Read the model definition and answer for the solid it produces. Units are mm, in the model's axes. A direction names the side the tool comes from. Give positions to 0.01 mm unless a question says otherwise; leave off trailing zeros. Order: outer loops, then holes, each group sorted by start corner. A loop starts at its lowest first (then second) coordinate and runs counter-clockwise, first axis right, second up. Notation, with made-up numbers: (56.25, 51) -> (67.25, 51) arc R7 cw to (67.25, 60) -> close; hole circle Ø9 at (79.5, -2.5). An arc over 180 degrees is marked (long way). One line per question, with ' | ' between items. Start each with the question number.
```python
from build123d import *

# Parameters (mm, degrees)
SKETCH1_W           = 51.225
SKETCH1_H           = 33.05
BOSS_EXTRUDE1_DEPTH = 6.35
SKETCH7_R           = 11.05
SKETCH7_R_2         = 3.556
CUT_EXTRUDE3_DEPTH  = 4.7625
SKETCH8_R           = 1.25
CUT_EXTRUDE4_DEPTH  = 15
FILLET3_R           = 5.08
CHAMFER2_SIZE       = 0.2


with BuildPart() as part:
    # Sketch1 → Boss-Extrude1 (new body)
    with BuildSketch(Plane.XY.offset(152.111703917)):
        with Locations((-7.6125, 2.525)):
            Rectangle(SKETCH1_W, SKETCH1_H)
    extrude(amount=-BOSS_EXTRUDE1_DEPTH)

    # Sketch7 → Cut-Extrude3 (cut)
    with BuildSketch(Plane.XY.offset(152.111703917)):
        Circle(SKETCH7_R)
        with Locations((-22.225, 0)):
            Circle(SKETCH7_R_2)
    extrude(amount=-CUT_EXTRUDE3_DEPTH, mode=Mode.SUBTRACT)

    # Sketch8 → Cut-Extrude4 (cut)
    with BuildSketch(Plane(origin=(0, 19.05, 0), x_dir=(1, 0, 0), z_dir=(0, 1, 0))):
        with Locations(Location((-29.725, -148.936703917, 0), (0, 0, 270))):
            Circle(SKETCH8_R)
        with Locations(Location((-14, -148.936703917, 0), (0, 0, 270))):
            Circle(SKETCH8_R)
        with Locations(Location((14.5, -148.936703917, 0), (0, 0, 270))):
            Circle(SKETCH8_R)
    extrude(amount=-CUT_EXTRUDE4_DEPTH, mode=Mode.SUBTRACT)

    # Fillet3
    fillet3_edges = [part.edges().sort_by_distance(p)[0] for p in [
        (18, -14, 148.936703917),
        (-33.225, -14, 148.936703917),
    ]]
    fillet(fillet3_edges, radius=FILLET3_R)

    # Chamfer2
    chamfer2_edges = [part.edges().sort_by_distance(p)[0] for p in [
        (-11.05, 0, 152.111703917),
        (-25.781, 0, 152.111703917),
        (-29.725, 19.05, 147.686703917),
        (-14, 19.05, 147.686703917),
        (14.5, 19.05, 147.686703917),
        (-7.6125, -14, 152.111703917),
        (18, 5.065, 152.111703917),
        (-31.737102448, -12.512102448, 152.111703917),
        (16.512102448, -12.512102448, 152.111703917),
        (-33.225, 5.065, 152.111703917),
    ]]
    chamfer(chamfer2_edges, length=CHAMFER2_SIZE)


solid = part.part
```
Q1. A cutting plane is placed at C-C, the plane y = 0. Determine the outline of the cut face in (x, z) (3 decimals), then the cut area to 3 significant figures.
Q2. A cutting plane is placed at D-D, the plane y = 17.5. Determine the outline of the cut face in (x, z) (3 decimals), then the cut area to 3 significant figures.
Q3. Determine the mould class of faces 4 (the flat face through (15, 4.05, 149)), 5 (the flat face through (-8, 19.05, 149)), 6 (the cylindrical face through (16.472, -12.551, 148.794)), 7 (the cylindrical face through (-14.48, 11.55, 150.09)) for opening direction X: pulls with the +X half, pulls with the -X half, needs draft (parallel to the pull), parting line crosses it, or undercut.
Q4. A cutting plane is placed at B-B, the plane z = 151. Determine the outline of the cut face in (x, y) (3 decimals), then the cut area to 3 significant figures.
Q5. Which of the six approach directions +Z, -Z, +X, -X, +Y, -Y give full straight-line access (tool end or side, diameter ignored) to faces 1 (the flat face through (-30, 4.05, 149)), 2 (the cylindrical face through (-31.78, -12.47, 148.79)), 3 (the cylindrical face through (-25.778, 0.156, 149.662))?
Q6. Given P1, Ø0.8, axis at x = -14, z = 148.5, coming from the +Y side; P2, Ø6.5, axis at x = -22.225, y = 0, coming from the +Z side; P3, Ø3, axis at x = -29, z = 149, coming from the +Y side, each flat-ended and moving along its own axis, determine where each tip first touches the part or whether it passes through.
Q7. A cutting plane is placed at A-A, the plane x = 0. Determine the outline of the cut face in (y, z), then the cut area to 3 significant figures.
Q8. Find the intervals of material crossed by line 1 (X direction, y = -2, z = 149.5) (1 decimal); line 2 (X direction, y = 17, z = 148.25) (3 decimals); line 3 (Y direction, x = -22, z = 150), in increasing order.
Geometry results:
1) outline: (-33.225, 145.762) -> (18, 145.762) -> (18, 151.912) -> (17.8, 152.112) -> (11.25, 152.112) -> (11.05, 151.912) -> (11.05, 147.349) -> (-11.05, 147.349) -> (-11.05, 151.912) -> (-11.25, 152.112) -> (-18.469, 152.112) -> (-18.669, 151.912) -> (-18.669, 147.349) -> (-25.781, 147.349) -> (-25.781, 151.912) -> (-25.981, 152.112) -> (-33.025, 152.112) -> (-33.225, 151.912) -> close | area: 186 mm²
2) outline: (-33.225, 145.762) -> (18, 145.762) -> (18, 151.912) -> (17.8, 152.112) -> (-33.025, 152.112) -> (-33.225, 151.912) -> close; hole circle Ø2.5 at (-29.725, 148.937); hole circle Ø2.5 at (-14, 148.937); hole circle Ø2.5 at (14.5, 148.937) | area: 311 mm²
3) face 4: undercut | face 5: needs draft | face 6: pulls with the +X half | face 7: undercut
4) outline: (-33.225, -8.92) arc R5.08 ccw to (-28.145, -14) -> (12.92, -14) arc R5.08 ccw to (18, -8.92) -> (18, 19.05) -> (-33.225, 19.05) -> close; hole circle Ø7.112 at (-22.225, 0); hole circle Ø22.1 at (0, 0) | area: 1,260 mm²
5) face 1: +Y | face 2: +Z, -Z, -X, -Y | face 3: +Z
6) P1: y = 4.05 | P2: z = 147.35 | P3: y = 19.05
7) outline: (-14, 145.76) -> (19.05, 145.76) -> (19.05, 152.11) -> (11.25, 152.11) -> (11.05, 151.91) -> (11.05, 147.35) -> (-11.05, 147.35) -> (-11.05, 151.91) -> (-11.25, 152.11) -> (-13.8, 152.11) -> (-14, 151.91) -> close | area: 105 mm²
8) line 1: -33.2 to -25.2, -19.3 to -10.9, 10.9 to 18 | line 2: -33.225 to -30.769, -28.681 to -15.044, -12.956 to 13.456, 15.544 to 18 | line 3: -14 to -3.55, 3.55 to 19.05
